Model file for the job. Use its own axes, mm. Face numbers are marked on the shaded views. A direction names the side the tool comes from. Give positions to 0.01 mm unless a question says otherwise; leave off trailing zeros. Loops run counter-clockwise (first coordinate to the right, second up) from the corner with the lowest first, then second, coordinate; pieces in that order, holes last. Notation, with made-up numbers: (-33.5, -9) - (-16.5, -9) arc R18 ccw to (-16.5, 11) - close; hole circle Ø10 at (87, -12.75). An arc over 180 degrees is marked (long way). Answer as CSV lines item,"result". Start each with the question number.
Item 1: Saw through at B-B on z = 14.5. Give the cut face in (x, y), plus the area to 3 significant figures.
Item 2: Saw through at A-A on x = -59. Give the cut face in (y, z).
Item 3: Saw through at C-C on y = -8. Give the cut face in (x, z), plus the area to 3 significant figures.
Item 4: Tool access for the marked faces 5 and 6: list every direction of +Z, -Z, +X, -X, +Y, -Y with a clear straight run to the whole face (end or side of a thin tool).
Item 5: Pin check, flat tips, straight feed: pin 1 (1 mm diameter, centred on x = 3.5, y = 1, fed in from +Z); pin 2 (4.5 mm diameter, centred on x = -97.5, y = -68.5, fed in from -Z). Stop position of each tip, or through.
Item 6: Pull direction X, two halves, no side cores. Call the marked faces 1, 2, 3 and 4: pulls with the +X half, pulls with the -X half, needs draft (parallel to the pull), parting line crosses it, or undercut.
Item 7: Drill centre lines: L1, parallel to X at y = 66, z = 51; L2, parallel to Y at x = -118.5, z = 59.25; L3, parallel to X at y = -66, z = 59.5. Where is each one in solid material? Low to high. Write a range as from..to.
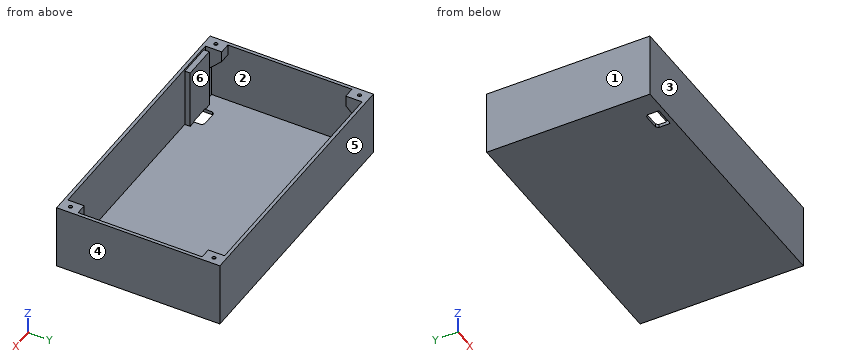
Autodesk Inventor part; units mm, degrees
ref_plane "YZ Plane" through (0, 0, 0) normal (1, 0, 0) x (0, 1, 0)
ref_plane "XZ Plane" through (0, 0, 0) normal (0, 1, 0) x (-1, 0, 0)
ref_plane "XY Plane" through (0, 0, 0) normal (0, 0, 1) x (1, 0, 0)
sketch "Sketch7" plane through (0, 0, 0) normal (0, 0, 1) x (1, 0, 0)
  line L0 (125, -75) -> (-125, -75)
  line L1 (-125, -75) -> (-125, 75)
  line L2 (-125, 75) -> (125, 75)
  line L3 (125, 75) -> (125, -75)
  line L4 (125, -75) -> (-125, 75) construction
  line L5 (-125, -75) -> (125, 75) construction
  point P0 (0, 0)
  dimension "d15" = 250
  dimension "d16" = 150
extrude "Box Outside" add sketch "Sketch7" along normal blind 60
sketch "Sketch8" plane through (0, 0, 60) normal (0, 0, 1) x (1, 0, 0)
  line L0 (-122, 72) -> (122, 72)
  line L1 (122, 72) -> (122, -72)
  line L2 (122, -72) -> (-122, -72)
  line L3 (-122, -72) -> (-122, 72)
  line L4 (125, 75) -> (-125, 75)
  line L5 (-125, 75) -> (-125, -75)
  line L6 (-125, -75) -> (125, -75)
  line L7 (125, -75) -> (125, 75)
  point P0 (0, 0)
  dimension "d19" = 3
  dimension "d20" = 3
  dimension "d21" = 3
  dimension "d22" = 3
extrude "Box Cut" cut sketch "Sketch8" against normal blind 57 contours L0 L1 L2 L3
sketch "Sketch9" plane through (-122, -72, 60) normal (0, 1, 0) x (1, 0, 0)
  line L0 (0, 0) -> (10, 0)
  line L1 (10, 0) -> (10, 25)
  line L2 (10, 25) -> (0, 25)
  line L3 (0, 25) -> (0, 0)
  point P0 (122, 60)
  dimension "d25" = 10
  dimension "d26" = 25
extrude "ScrewHole Box LB" add sketch "Sketch9" along normal blind 15
sketch "Sketch10" plane through (-122, -72, 3) normal (0, 1, 0) x (1, 0, 0)
  line L0 (244, -57) -> (244, 0)
  line L1 (244, -57) -> (234, -57)
  line L2 (234, -57) -> (234, -32)
  line L3 (234, -32) -> (244, -32)
  line L4 (244, -32) -> (244, -57)
  point P0 (122, 3)
  dimension "d29" = 10
  dimension "d30" = 25
extrude "ScrewHole Box RB" add sketch "Sketch10" along normal blind 15
sketch "Sketch11" plane through (-122, 72, 60) normal (0, -1, 0) x (1, 0, 0)
  line L0 (0, 0) -> (244, 0)
  line L1 (0, 0) -> (10, 0)
  line L2 (10, 0) -> (10, -25)
  line L3 (10, -25) -> (0, -25)
  line L4 (0, -25) -> (0, 0)
  point P0 (122, -60)
  dimension "d33" = 10
  dimension "d34" = 25
extrude "ScrewHole Box LU" add sketch "Sketch11" along normal blind 15
sketch "Sketch13" plane through (122, -72, 3) normal (-1, 0, 0) x (0, 0, 1)
  line L0 (57, 144) -> (0, 144)
  line L1 (57, 144) -> (32, 144)
  line L2 (32, 144) -> (32, 129)
  line L3 (32, 129) -> (57, 129)
  line L4 (57, 129) -> (57, 144)
  point P0 (-3, 72)
  dimension "d37" = 25
  dimension "d38" = 15
extrude "ScrewHole Box RU" add sketch "Sketch13" along normal blind 10
sketch "Sketch27" plane through (0, 0, 60) normal (0, 0, 1) x (1, 0, 0)
  line L0 (-112, -72) -> (-112, -57)
  line L1 (-125, 75) -> (-125, -75)
  line L2 (-112, -57) -> (-125, -57)
  line L3 (-125, -57) -> (-125, -75)
  line L4 (-125, -75) -> (-112, -75)
  line L5 (-112, -75) -> (-112, -57)
  line L6 (-112, -57) -> (-125, -75)
  line L7 (-112, -75) -> (-125, -57)
  circle A0 centre (-118.5, -66) radius 2.4
  point P0 (0, 0)
  dimension "d84" = 4.8
extrude "Outside ScrewHole LB" cut sketch "Sketch27" against normal blind 26 contours A0 L7 L6 | L6 L7 A0 | A0 L6 L7 | L7 L6 A0
sketch "Sketch29" plane through (0, 0, 60) normal (0, 0, 1) x (1, 0, 0)
  line L0 (-112, -72) -> (-112, -57)
  line L1 (-125, -75) -> (125, -75)
  line L2 (-112, -57) -> (-125, -57)
  line L3 (-125, -57) -> (-125, -75)
  line L4 (-125, -75) -> (-112, -75)
  line L5 (-112, -75) -> (-112, -57)
  line L6 (-112, -57) -> (-125, -75)
  circle A0 centre (-118.5, -66) radius 2.4
  point P0 (0, 0)
extrude "ScrewRibbon LB" add sketch "Sketch29" against normal blind 2 contours A0 L6 | L6 A0
sketch "Sketch30" plane through (0, 0, 60) normal (0, 0, 1) x (1, 0, 0)
  line L0 (-122, -57) -> (-112, -57)
  line L1 (-125, -75) -> (125, -75)
  line L2 (-112, -57) -> (-125, -57)
  line L3 (-125, -57) -> (-125, -75)
  line L4 (-125, -75) -> (-112, -75)
  line L5 (-112, -75) -> (-112, -57)
  line L6 (-112, -57) -> (-125, -75)
  circle A0 centre (-118.5, -66) radius 1.7
  point P0 (0, 0)
  dimension "d92" = 3.4
extrude "Inside ScrewHole LB" cut sketch "Sketch30" against normal blind 24 contours A0 L6 | L6 A0
sketch "Sketch31" plane through (0, 0, 60) normal (0, 0, 1) x (1, 0, 0)
  line L0 (-125, 75) -> (-125, -75)
  line L1 (-112, 57) -> (-122, 57)
  line L2 (-125, 75) -> (-112, 75)
  line L3 (-112, 75) -> (-112, 57)
  line L4 (-112, 57) -> (-125, 57)
  line L5 (-125, 57) -> (-125, 75)
  line L6 (-125, 75) -> (-112, 57)
  circle A0 centre (-118.5, 66) radius 2.4
  point P0 (0, 0)
  dimension "d95" = 4.8
extrude "Outside ScrewHole LU" cut sketch "Sketch31" against normal blind 24 contours A0 L6 | L6 A0
sketch "Sketch32" plane through (0, 0, 60) normal (0, 0, 1) x (1, 0, 0)
  line L0 (-122, 57) -> (-112, 57)
  line L1 (-125, 75) -> (-125, -75)
  line L2 (-112, 57) -> (-125, 57)
  line L3 (-125, 57) -> (-125, 75)
  line L4 (-125, 75) -> (-112, 75)
  line L5 (-112, 75) -> (-112, 57)
  line L6 (-112, 75) -> (-125, 57)
  circle A0 centre (-118.5, 66) radius 2.4
  point P0 (0, 0)
  dimension "d98" = 4.8
extrude "ScrewRibbon LU" add sketch "Sketch32" against normal blind 2 contours A0 L6 | L6 A0
sketch "Sketch33" plane through (0, 0, 60) normal (0, 0, 1) x (1, 0, 0)
  line L0 (125, 75) -> (-125, 75)
  line L1 (-112, 57) -> (-122, 57)
  line L2 (-125, 75) -> (-112, 75)
  line L3 (-112, 75) -> (-112, 57)
  line L4 (-112, 57) -> (-125, 57)
  line L5 (-125, 57) -> (-125, 75)
  line L6 (-125, 75) -> (-112, 57)
  circle A0 centre (-118.5, 66) radius 1.7
  point P0 (0, 0)
  dimension "d101" = 3.4
extrude "Inside ScrewHole LU" cut sketch "Sketch33" against normal blind 21.75 contours A0 L6 | L6 A0
sketch "Sketch34" plane through (0, 0, 60) normal (0, 0, 1) x (1, 0, 0)
  line L0 (112, 57) -> (112, 72)
  line L1 (125, 75) -> (-125, 75)
  line L2 (112, 57) -> (125, 57)
  line L3 (125, 57) -> (125, 75)
  line L4 (125, 75) -> (112, 75)
  line L5 (112, 75) -> (112, 57)
  line L6 (125, 75) -> (112, 57)
  circle A0 centre (118.5, 66) radius 2.4
  point P0 (0, 0)
  dimension "d104" = 4.8
extrude "Outside ScrewHole RU" cut sketch "Sketch34" against normal blind 37 contours A0 L6 | L6 A0
sketch "Sketch35" plane through (0, 0, 60) normal (0, 0, 1) x (1, 0, 0)
  line L0 (125, -75) -> (125, 75)
  line L1 (122, 57) -> (112, 57)
  line L2 (125, 75) -> (112, 75)
  line L3 (112, 75) -> (112, 57)
  line L4 (112, 57) -> (125, 57)
  line L5 (125, 57) -> (125, 75)
  line L6 (125, 75) -> (-125, 75)
  line L7 (125, 75) -> (112, 57)
  circle A0 centre (118.5, 66) radius 2.4
  point P0 (0, 0)
  dimension "d107" = 4.8
extrude "ScrewRibbon RU" add sketch "Sketch35" against normal blind 2 contours A0 L7 | L7 A0
sketch "Sketch36" plane through (0, 0, 60) normal (0, 0, 1) x (1, 0, 0)
  line L0 (122, 57) -> (112, 57)
  line L1 (125, -75) -> (125, 75)
  line L2 (112, 57) -> (125, 57)
  line L3 (125, 57) -> (125, 75)
  line L4 (125, 75) -> (112, 75)
  line L5 (112, 75) -> (112, 57)
  line L6 (112, 57) -> (125, 75)
  circle A0 centre (118.5, 66) radius 2.4
  circle A1 centre (118.5, 66) radius 1.7
  point P0 (0, 0)
  dimension "d110" = 3.4
extrude "Inside ScrewHole RU" cut sketch "Sketch36" against normal blind 20 contours A1 L6 | L6 A1
sketch "Sketch37" plane through (0, 0, 60) normal (0, 0, 1) x (1, 0, 0)
  line L0 (125, -75) -> (125, 75)
  line L1 (112, -72) -> (112, -57)
  line L2 (125, -75) -> (112, -75)
  line L3 (112, -75) -> (112, -57)
  line L4 (112, -57) -> (125, -57)
  line L5 (125, -57) -> (125, -75)
  line L6 (112, -75) -> (125, -57)
  circle A0 centre (118.5, -66) radius 2.4
  point P0 (0, 0)
  dimension "d113" = 4.8
extrude "Outside ScrewHole RB" cut sketch "Sketch37" against normal blind 27.5 contours A0 L6 | L6 A0
sketch "Sketch38" plane through (0, 0, 60) normal (0, 0, 1) x (1, 0, 0)
  line L0 (122, -57) -> (112, -57)
  line L1 (125, -75) -> (125, 75)
  line L2 (112, -57) -> (125, -57)
  line L3 (125, -57) -> (125, -75)
  line L4 (125, -75) -> (112, -75)
  line L5 (112, -75) -> (112, -57)
  line L6 (125, -57) -> (112, -75)
  circle A0 centre (118.5, -66) radius 2.4
  point P0 (0, 0)
  dimension "d116" = 4.8
extrude "ScrewRibbon RB" add sketch "Sketch38" against normal blind 2 contours A0 L6 | L6 A0
sketch "Sketch39" plane through (0, 0, 60) normal (0, 0, 1) x (1, 0, 0)
  line L0 (112, -72) -> (112, -57)
  line L1 (125, -75) -> (125, 75)
  line L2 (112, -57) -> (125, -57)
  line L3 (125, -57) -> (125, -75)
  line L4 (125, -75) -> (112, -75)
  line L5 (112, -75) -> (112, -57)
  line L6 (112, -75) -> (125, -57)
  circle A0 centre (118.5, -66) radius 2.4
  circle A1 centre (118.5, -66) radius 1.7
  point P0 (0, 0)
  dimension "d119" = 3.4
extrude "Inside ScrewHole RB" cut sketch "Sketch39" against normal blind 20 contours A1 L6 | L6 A1
sketch "Sketch42" plane through (-122, -72, 3) normal (0, 1, 0) x (1, 0, 0)
  line L0 (244, 0) -> (0, 0)
  line L1 (12.5963, 0) -> (43.5963, 0)
  line L2 (43.5963, 0) -> (43.5963, -55)
  line L3 (43.5963, -55) -> (12.5963, -55)
  line L4 (12.5963, -55) -> (12.5963, 0)
  point P0 (122, 3)
  point P1 (43.5963, 0)
  dimension "d134" = 31
  dimension "d135" = 55
extrude "ESPHolder" add sketch "Sketch42" along normal blind 5
sketch "Sketch43" plane through (0, 0, 3) normal (0, 0, 1) x (1, 0, 0)
  line L0 (-109.4037, -67) -> (-78.4037, -67)
  line L1 (-99.1037, -67) -> (-88.7037, -67)
  line L2 (-88.7037, -67) -> (-88.7037, -62.5)
  line L3 (-88.7037, -62.5) -> (-99.1037, -62.5)
  line L4 (-99.1037, -62.5) -> (-99.1037, -67)
  line L5 (-78.4037, -67) -> (-109.4037, -67)
  line L6 (-109.4037, -67) -> (-109.4037, -51.7804)
  line L7 (-109.4037, -51.7804) -> (-78.4037, -51.7804)
  line L8 (-78.4037, -51.7804) -> (-78.4037, -67)
  point P0 (0, 0)
  dimension "d138" = 10.3
  dimension "d139" = 10.3
  dimension "d140" = 4.5
extrude "PortHole" cut sketch "Sketch43" against normal through all contours L4 L3 L2 L0
sketch "Sketch44" plane through (0, 0, 0) normal (0, 0, -1) x (-1, 0, 0)
  line L0 (84.7037, -58.5) -> (103.1037, -58.5)
  line L1 (103.1037, -58.5) -> (103.1037, -71)
  line L2 (103.1037, -71) -> (84.7037, -71)
  line L3 (84.7037, -71) -> (84.7037, -58.5)
  line L4 (88.7037, -62.5) -> (99.1037, -62.5)
  line L5 (99.1037, -67) -> (88.7037, -67)
  line L6 (99.1037, -62.5) -> (99.1037, -67)
  line L7 (88.7037, -67) -> (88.7037, -62.5)
  point P0 (0, 0)
  dimension "d143" = 4
  dimension "d144" = 4
  dimension "d145" = 4
  dimension "d146" = 4
extrude "Extrusion29" cut sketch "Sketch44" against normal blind 4
chamfer "Chamfer1" distance 15 angle 45 1 edges at (-117, -57, 35)
chamfer "Chamfer2" distance 15 angle 45 1 edges at (-117, 57, 35)
chamfer "Chamfer3" distance 15 angle 45 1 edges at (117, 57, 35)
chamfer "Chamfer4" distance 15 angle 45 1 edges at (117, -57, 35)
chamfer "Chamfer5" distance 2 angle 45 2 edges at (-84.7037, -58.5, 1.5) (-103.1037, -58.5, 1.5)
properties part number "Box2"
Responses:
1,outline,"(-125, -75) - (125, -75) - (125, 75) - (-125, 75) - close; hole (-122, -72) - (-109.4, -72) - (-109.4, -67) - (-78.4, -67) - (-78.4, -72) - (122, -72) - (122, 72) - (-122, 72) - close"
1,area,"2,520 mm2"
2,outline,"(-75, 0) - (75, 0) - (75, 60) - (72, 60) - (72, 3) - (-72, 3) - (-72, 60) - (-75, 60) - close"
3,outline,"(-125, 0) - (125, 0) - (125, 60) - (122, 60) - (122, 3) - (-122, 3) - (-122, 60) - (-125, 60) - close"
3,area,"1,090 mm2"
4,face 5,"+Z, -Z, +X, -X, +Y"
4,face 6,"+Z"
5,pin 1,"z = 3"
5,pin 2,"z = 4"
6,face 1,"pulls with the -X half"
6,face 2,"undercut"
6,face 3,"needs draft"
6,face 4,"pulls with the +X half"
7,L1,"-125..-120.9, -116.1..-112, 112..116.1, 120.9..125"
7,L2,"-75..-67.7, -64.3..-57, 57..64.3, 67.7..75"
7,L3,"-125..-120.2, -116.8..-112, 112..116.8, 120.2..125"
